from build123d import *

# Parameters (mm, degrees)
SKETCH1_W           = 40
SKETCH1_H           = 83.2
SKETCH1_W_2         = 15.916627574
SKETCH1_H_2         = 8.6
BOSS_EXTRUDE1_DEPTH = 48
CHAMFER1_SIZE       = 48
CHAMFER1_SIZE_2     = 3.356486973
BOSS_EXTRUDE2_START = 48
SKETCH1_3_W         = 15.916627574
SKETCH1_3_H         = 8.6
BOSS_EXTRUDE2_DEPTH = 3
FILLET1_R           = 4


with BuildPart() as part:
    # Sketch1 → Boss-Extrude1 (new body)
    # profile 1 of 4: a face of its own
    with BuildSketch(Plane(origin=(0, 0, 0), x_dir=(1, 0, 0), z_dir=(0, 1, 0))):
        Rectangle(SKETCH1_W, SKETCH1_H)
        Polygon((8.620526076, 6.8), (0, 22.5), (-8.620526076, 6.8), align=None, mode=Mode.SUBTRACT)
        Rectangle(SKETCH1_W_2, SKETCH1_H_2, mode=Mode.SUBTRACT)
        Polygon((-8.620526076, -6.8), (0, -22.5), (8.620526076, -6.8), align=None, mode=Mode.SUBTRACT)
    # profile 2 of 4: a face of its own
    with BuildSketch(Plane(origin=(0, 0, 0), x_dir=(1, 0, 0), z_dir=(0, 1, 0))):
        Polygon((-8.620526076, 6.8), (8.620526076, 6.8), (0, 22.5), align=None)
    # profile 3 of 4: a face of its own
    with BuildSketch(Plane(origin=(0, 0, 0), x_dir=(1, 0, 0), z_dir=(0, 1, 0))):
        Rectangle(SKETCH1_W_2, SKETCH1_H_2)
    # profile 4 of 4: a face of its own
    with BuildSketch(Plane(origin=(0, 0, 0), x_dir=(1, 0, 0), z_dir=(0, 1, 0))):
        Polygon((-8.620526076, -6.8), (8.620526076, -6.8), (0, -22.5), align=None)
    extrude(amount=BOSS_EXTRUDE1_DEPTH)

    # Chamfer1
    # the kernel refuses this chamfer: 48, 3.356486973 mm, written as the material it takes off along each edge
    with BuildSketch(Plane(origin=(144.788756649, 48, 41.6), x_dir=(0, -0.999996400257939, 0.002683183028377395), z_dir=(-1, 0, 0)), Plane(origin=(-144.788756649, 48, -41.6), x_dir=(0, -0.999996400257939, -0.002683183028377395), z_dir=(1, 0, 0))) as chamfer1_piece_1:
        Polygon((CHAMFER1_SIZE * 0.999996400258, -CHAMFER1_SIZE * 0.00268318302838), (-CHAMFER1_SIZE_2 * 0.00268318302861, -CHAMFER1_SIZE_2 * 0.999996400344), (0, 0), align=None)
    extrude(amount=289.577513297, mode=Mode.SUBTRACT)
    with BuildSketch(Plane(origin=(-20, 48, 166.388756649), x_dir=(0.8766829747338886, 0.4810685624853697, 0), z_dir=(0, 0, -1))) as chamfer1_piece_2:
        Polygon((CHAMFER1_SIZE_2 * 0.876682974809, CHAMFER1_SIZE_2 * 0.481068562527), (-CHAMFER1_SIZE * 0.481068562485, CHAMFER1_SIZE * 0.876682974734), (0, 0), align=None)
    extrude(amount=332.777513297, mode=Mode.SUBTRACT)
    with BuildSketch(Plane(origin=(20, 48, -166.388756649), x_dir=(0.002683183028377466, -0.999996400257939, 0), z_dir=(0, 0, 1))) as chamfer1_piece_3:
        Polygon((CHAMFER1_SIZE * 0.999996400258, -CHAMFER1_SIZE * 0.00268318302838), (-CHAMFER1_SIZE_2 * 0.00268318302861, -CHAMFER1_SIZE_2 * 0.999996400344), (0, 0), align=None)
    extrude(amount=332.777513297, mode=Mode.SUBTRACT)

    # Sketch1<3> → Boss-Extrude2 (add)
    with BuildSketch(Plane(origin=(0, 0, 0), x_dir=(1, 0, 0), z_dir=(0, 1, 0)).offset(BOSS_EXTRUDE2_START)):
        Polygon((-8.620526076, 6.8), (8.620526076, 6.8), (0, 22.5), align=None)
        Rectangle(SKETCH1_3_W, SKETCH1_3_H)
        Polygon((-8.620526076, -6.8), (8.620526076, -6.8), (0, -22.5), align=None)
    extrude(amount=BOSS_EXTRUDE2_DEPTH)

    # Fillet1
    fillet1_edges = [part.edges().sort_by_distance(p)[0] for p in [
        (16.643513027, 48, 0),
        (0, 48, -38.243513027),
        (-16.643513027, 48, 0),
        (0, 48, 38.243513027),
        (-18.321756513, 24, -39.921756513),
        (18.321756513, 24, -39.921756513),
        (-18.321756513, 24, 39.921756513),
        (18.321756513, 24, 39.921756513),
    ]]
    fillet(fillet1_edges, radius=FILLET1_R)


solid = part.part
Here's how the part is built. I have some questions about the finished solid (model axes, mm). A direction names the side the tool comes from. Coordinates: 2 decimals unless noted, no trailing zeros. Order: outer loops, then holes, each group sorted by start corner. A loop starts at its lowest first (then second) coordinate and runs counter-clockwise, first axis right, second up. Notation, with made-up numbers: M -8.75,-26.75 L 36.25,-26.75 A28 ccw 36.25,4.25 Z; hole C 27,53 d6. An arc over 180 degrees is marked long. Answer as CSV lines item,"result". Start each with the question number.
1. On a 3-axis mill with a long thin cutter (end or side, diameter ignored), from which of +Z, -Z, +X, -X, +Y, -Y can I reach the whole of each face in a straight line? I mean faces 1 (the flat face through (0, 49, -4.3)), 2 (the flat face through (4.37, 49.48, 14.54)), 3 (the flat face through (7.958, 49, 0)). Say none if no direction works.
2. I want a section at D-D, the plane x = 12. Write out the boundary of the cut face in (y, z), and give its area (3 significant figures).
3. I want a section at B-B, the plane x = -5. Write out the boundary of the cut face in (y, z), and give its area (3 significant figures).
4. I want a section at C-C, the plane z = -11. Write out the boundary of the cut face in (x, y), and give its area (3 significant figures).
5. We'd pull the mould along Z, two halves only. Please class faces 4 (the flat face through (-4.25, 49.48, 14.76)), 5 (the cylindrical face through (15.67, 46.9, 0.48)), 6 (the flat face through (0, 49, -6.8)): released by +Z, released by -Z, zero draft, split by the parting line, or undercut.
6. I want a section at A-A, the plane z = 25. Write out the boundary of the cut face in (x, y), and give its area (3 significant figures).
7. I need wall thicknesses on line 1 (Y direction, x = 0.5, z = -32); line 2 (Z direction, x = -14, y = 46.5); line 3 (X direction, y = 45, z = 27.5). Which ranges of each line are inside material? Lowest first, please. Write a range as [from, to].
8. For pin 1 (0.9 mm diameter, centred on x = 3.5, y = 49, fed in from -Z); pin 2 (1.5 mm diameter, centred on y = 50, z = -1.5, fed in from -X); pin 3 (2 mm diameter, centred on y = 8, z = -15, fed in from +X), each with a flat end and sliding along its axis, tell me the tip position at first contact or that it passes through.
Recorded:
1,face 1,"+X, -X, +Y"
1,face 2,"+Z, +X, +Y"
1,face 3,"+X, +Y"
2,outline,"M 0,-41.6 L 44.28,-38.5 A4 ccw 48,-34.51 L 48,34.51 A4 ccw 44.28,38.5 L 0,41.6 Z"
2,area,"3,830 mm2"
3,outline,"M 0,-41.6 L 44.28,-38.5 A4 ccw 48,-34.51 L 48,-13.39 L 51,-13.39 L 51,-6.8 L 48,-6.8 L 48,-4.3 L 51,-4.3 L 51,4.3 L 48,4.3 L 48,6.8 L 51,6.8 L 51,13.39 L 48,13.39 L 48,34.51 A4 ccw 44.28,38.5 L 0,41.6 Z"
3,area,"3,890 mm2"
4,outline,"M -20,0 L 20,0 L 16.9,44.28 A4 ccw 12.91,48 L 6.31,48 L 6.31,51 L -6.31,51 L -6.31,48 L -12.91,48 A4 ccw -16.9,44.28 Z"
4,area,"1,790 mm2"
5,face 4,"released by +Z"
5,face 5,"zero draft"
5,face 6,"undercut"
6,outline,"M -20,0 L 20,0 L 16.9,44.28 A4 ccw 12.91,48 L -12.91,48 A4 ccw -16.9,44.28 Z"
6,area,"1,750 mm2"
7,line 1,"y = [0, 48]"
7,line 2,"z = [-37.44, 37.44]"
7,line 3,"x = [-16.79, 16.79]"
8,pin 1,"stops at z = -16.95"
8,pin 2,"stops at x = -7.96"
8,pin 3,"stops at x = 19.51"
